Source: CAD feature listing. Evaluate the final solid. Frame: model axes, mm. A direction names the side the tool comes from. Coordinates: 2 decimals unless noted, no trailing zeros. Write each loop counter-clockwise with the first axis right and the second up, starting at its lowest first coordinate (ties: lowest second). Pieces come first, ordered by that corner, then holes. Notation, with made-up numbers: (-12, 36.5) - (33, 36.5) arc R15 cw to (33, 58.5) - close; hole circle Ø11 at (30.25, 40.25). An arc over 180 degrees is marked (long way). One line per item, written item: value.
from build123d import *

# Parameters (mm, degrees)
EXTRUDE_1_DEPTH     = 3
EXTRUDE_2_DEPTH     = 3
SKETCH_2_R          = 1.25
CUT_EXTRUDE_1_DEPTH = 3
SKETCH_3_R          = 1.6
CUT_EXTRUDE_2_DEPTH = 3
FILLET_1_R          = 2


with BuildPart() as part:
    # 草图1 → 凸台-拉伸1 (new body)
    with BuildSketch(Plane(origin=(0, 0, 0), x_dir=(1, 0, 0), z_dir=(0, 1, 0))):
        with BuildLine():
            Line((-18, 25), (18, 25))
            ThreePointArc((18, 25), (19.414213562, 24.414213562), (20, 23))
            Line((20, 23), (20, -23))
            ThreePointArc((20, -23), (19.414213562, -24.414213562), (18, -25))
            Line((18, -25), (-18, -25))
            ThreePointArc((-18, -25), (-19.414213562, -24.414213562), (-20, -23))
            Line((-20, -23), (-20, 23))
            ThreePointArc((-20, 23), (-19.414213562, 24.414213562), (-18, 25))
        make_face()
    extrude(amount=EXTRUDE_1_DEPTH)

    # 草图4 → 凸台-拉伸2 (add)
    with BuildSketch(Plane(origin=(0, 3, 0), x_dir=(1, 0, 0), z_dir=(0, 1, 0))):
        with BuildLine():
            Line((-28, -11), (28, -11))
            ThreePointArc((28, -11), (29.414213562, -11.585786438), (30, -13))
            Line((30, -13), (30, -17))
            ThreePointArc((30, -17), (29.414213562, -18.414213562), (28, -19))
            Line((28, -19), (-28, -19))
            ThreePointArc((-28, -19), (-29.414213562, -18.414213562), (-30, -17))
            Line((-30, -17), (-30, -13))
            ThreePointArc((-30, -13), (-29.414213562, -11.585786438), (-28, -11))
        make_face()
    extrude(amount=-EXTRUDE_2_DEPTH)

    # 草图2 → 切除-拉伸1 (cut)
    with BuildSketch(Plane(origin=(0, 3, 0), x_dir=(1, 0, 0), z_dir=(0, 1, 0))):
        with Locations(Location((-25.1, -15, 0), (0, 0, 270))):
            Circle(SKETCH_2_R)
        with Locations(Location((-15.2, 8.6, 0), (0, 0, 270))):
            Circle(SKETCH_2_R)
        with Locations(Location((15.2, 8.6, 0), (0, 0, 90))):
            Circle(SKETCH_2_R)
        with Locations(Location((25.1, -15, 0), (0, 0, 90))):
            Circle(SKETCH_2_R)
    extrude(amount=-CUT_EXTRUDE_1_DEPTH, mode=Mode.SUBTRACT)

    # 草图3 → 切除-拉伸2 (cut)
    with BuildSketch(Plane(origin=(0, 3, 0), x_dir=(1, 0, 0), z_dir=(0, 1, 0))):
        with Locations(Location((-17, 22, 0), (0, 0, 270))):
            Circle(SKETCH_3_R)
        with Locations(Location((-17, -22, 0), (0, 0, 90))):
            Circle(SKETCH_3_R)
        with Locations(Location((17, -22, 0), (0, 0, 270))):
            Circle(SKETCH_3_R)
        with Locations(Location((17, 22, 0), (0, 0, 90))):
            Circle(SKETCH_3_R)
    extrude(amount=-CUT_EXTRUDE_2_DEPTH, mode=Mode.SUBTRACT)

    # 圆角1
    fillet_1_edges = [part.edges().sort_by_distance(p)[0] for p in [
        (-20, 1.5, 11),
        (20, 1.5, 11),
        (-20, 1.5, 19),
        (20, 1.5, 19),
    ]]
    fillet(fillet_1_edges, radius=FILLET_1_R)


solid = part.part
1) Reachability of faces 1 (the flat face through (20, 1, 22)), 2 (the flat face through (20, 1, -7)), 3 (the flat face through (-20, 1, -7)) from +Z, -Z, +X, -X, +Y, -Y: full face, straight path, thin tool, end or side. Return the list, or none.
Values found:
face 1: +Z, +X, +Y, -Y
face 2: -Z, +X, +Y, -Y
face 3: -Z, -X, +Y, -Y
2) Draft query along X for faces 4 (the cylindrical face through (-19.43, 1.48, -24.4)), 5 (the cylindrical face through (16.42, 1.52, -8.33)), 6 (the flat face through (30, 2, 15)). Return one class per face: released by +X, released by -X, zero draft, split by the parting line, or undercut.
Values found:
face 4: released by -X
face 5: undercut
face 6: released by +X
3) Section query B-B on x = -25.1. Output: boundary loops of the cut face in (y, z), then the cut area to 3 significant figures.
Values found:
outline: (0, 11) - (3, 11) - (3, 13.75) - (0, 13.75) - close; (0, 16.25) - (3, 16.25) - (3, 19) - (0, 19) - close
area: 16.5 mm2
4) Section query D-D on z = 22. Output: boundary loops of the cut face in (x, y).
Values found:
outline: (-20, 0) - (-18.6, 0) - (-18.6, 3) - (-20, 3) - close; (-15.4, 0) - (15.4, 0) - (15.4, 3) - (-15.4, 3) - close; (18.6, 0) - (20, 0) - (20, 3) - (18.6, 3) - close
5) Section query C-C on y = 2.2. State how many separate pieces and enclosed holes the cut face has, then the cut area to 3 significant figures.
Values found:
separate pieces: 1
enclosed holes: 8
area: 2,100 mm2
6) Section query A-A on z = -8.6. Output: boundary loops of the cut face in (x, y), then the cut area to 3 significant figures.
Values found:
outline: (-20, 0) - (-16.45, 0) - (-16.45, 3) - (-20, 3) - close; (-13.95, 0) - (13.95, 0) - (13.95, 3) - (-13.95, 3) - close; (16.45, 0) - (20, 0) - (20, 3) - (16.45, 3) - close
area: 105 mm2
7) Material intervals for line 1 (X direction, y = 1.85, z = -22); line 2 (X direction, y = 1.05, z = -8.6); line 3 (Z direction, x = 15.2, y = 2.35), sorted ascending.
Values found:
line 1: -20 to -18.6, -15.4 to 15.4, 18.6 to 20
line 2: -20 to -16.45, -13.95 to 13.95, 16.45 to 20
line 3: -25 to -9.85, -7.35 to 25
8) Contact query for flat-ended pins moving along their axis: P1, Ø0.9, axis at x = 24.5, y = 1, coming from the -Z side; P2, Ø1, axis at y = 1, z = 22, coming from the -X side; P3, Ø0.9, axis at x = -25.5, y = 1.5, coming from the +Z side. Output: stop coordinate, or through.
Values found:
P1: z = 11
P2: x = -20
P3: z = 19
